Could you check a few things on this drawing? It's one solid part, dimensions in mm from its lowest x, y, z. Give positions to 0.01 mm unless a question says otherwise; leave off trailing zeros. Write each loop counter-clockwise with the first axis right and the second up, starting at its lowest first coordinate (ties: lowest second). Pieces come first, ordered by that corner, then holes. Notation, with made-up numbers: (47.25, 65) - (95.25, 65) arc R29 cw to (95.25, 100) - close; hole circle Ø10 at (61.25, -33.5). An arc over 180 degrees is marked (long way). One line per item, written item: value. Start each with the question number.
1) Please list where these lines run through material, in increasing order: L1, parallel to X at y = 50.7, z = 0.8; L2, parallel to Y at x = 14, z = 1.05. Write a range as [from, to].
2) Imagine slicing it at D-D on y = 43.5. Write out the boundary of the cut face in (x, z), plus the area to 3 significant figures.
3) Imagine slicing it at A-A on y = 35.5. Write out the boundary of the cut face in (x, z).
4) I'm going to push a flat-ended pin straight in: P1, Ø0.5, axis at y = 44.5, z = 0.5, coming from the +X side. Where does the tip first touch, or does it pass through?
5) Imagine slicing it at B-B on z = 0.85. Write out the boundary of the cut face in (x, y), plus the area to 3 significant figures.
6) Imagine slicing it at C-C on y = 50.7. Write out the boundary of the cut face in (x, z), plus the area to 3 significant figures.
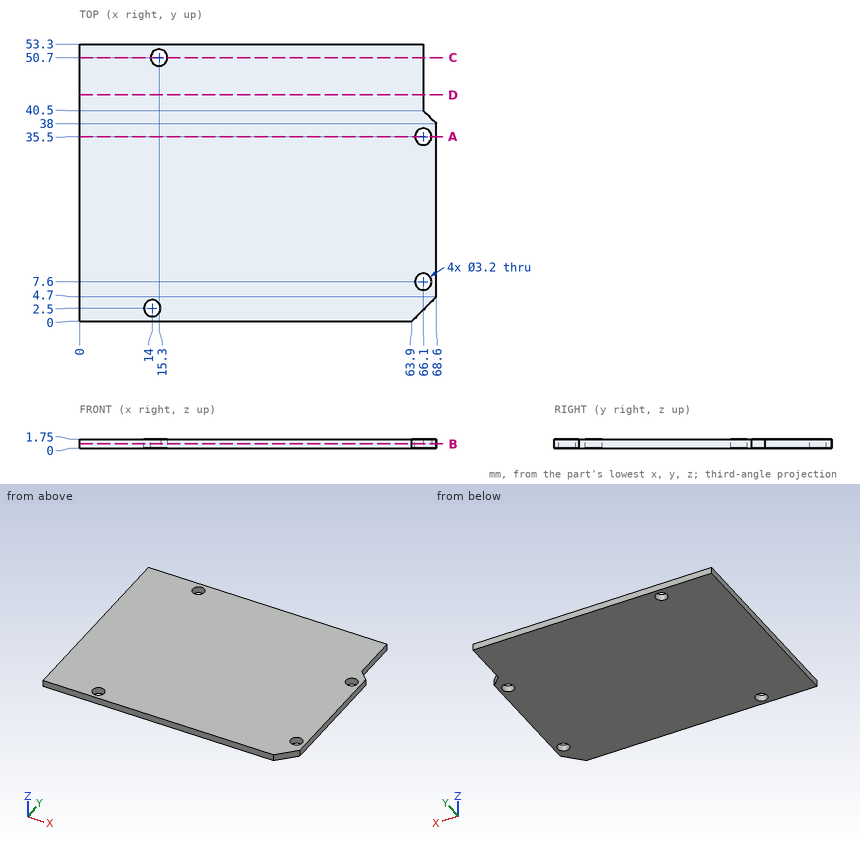
Numbers:
1. L1: [0, 13.7], [16.9, 66.1]
1. L2: [0, 0.9], [4.1, 49.77], [51.63, 53.3]
2. outline: (0, 0) - (66.1, 0) - (66.1, 1.75) - (0, 1.75) - close
2. area: 116 mm^2
3. outline: (0, 0) - (64.5, 0) - (64.5, 1.75) - (0, 1.75) - close; (67.7, 0) - (68.6, 0) - (68.6, 1.75) - (67.7, 1.75) - close
4. P1: x = 66.1
5. outline: (0, 0) - (63.9, 0) - (68.6, 4.7) - (68.6, 38) - (66.1, 40.5) - (66.1, 53.3) - (0, 53.3) - close; hole circle Ø3.2 at (14, 2.5); hole circle Ø3.2 at (15.3, 50.7); hole circle Ø3.2 at (66.1, 7.6); hole circle Ø3.2 at (66.1, 35.5)
5. area: 3,580 mm^2
6. outline: (0, 0) - (13.7, 0) - (13.7, 1.75) - (0, 1.75) - close; (16.9, 0) - (66.1, 0) - (66.1, 1.75) - (16.9, 1.75) - close
6. area: 110 mm^2
